from build123d import *

# Parameters (mm, degrees)
F1_DEPTH    = 1
F2_DEPTH    = 9
F2_TAPER    = 27
F3_T1_DEPTH = 17.6431556895
F3_T3_DEPTH = 17.6431556895
F3_T5_DEPTH = 17.6431556895
F3_T7_DEPTH = 17.6431556895
F4_R        = 18
F5_DEPTH    = 6
F5_TAPER    = 27
F6_R        = 3.05
F7_DEPTH    = 4.0010001


# Not quite as in the source:
# - a fillet or chamfer that OpenCascade refuses, or shapes differently, is made with other operations: its cross-section is extruded or revolved along the edge and cut away or added


with BuildPart() as f1:
    # F0 (on Top) → F1 (new body)
    with BuildSketch(Plane.XY):
        with BuildLine():
            Line((-17, -21), (17, -21))
            ThreePointArc((17, -21), (19.8284271247, -19.8284271247), (21, -17))
            Line((21, -17), (21, 17))
            ThreePointArc((21, 17), (19.8284271247, 19.8284271247), (17, 21))
            Line((17, 21), (-17, 21))
            ThreePointArc((-17, 21), (-19.8284271247, 19.8284271247), (-21, 17))
            Line((-21, 17), (-21, -17))
            ThreePointArc((-21, -17), (-19.8284271247, -19.8284271247), (-17, -21))
        make_face()
    extrude(amount=F1_DEPTH)

    # F1_face (on face) → F2 (join)
    with BuildSketch(Plane.XY.offset(1)):
        with BuildLine():
            Line((-17, -21), (17, -21))
            ThreePointArc((17, -21), (19.8284271247, -19.8284271247), (21, -17))
            Line((21, -17), (21, 17))
            ThreePointArc((21, 17), (19.8284271247, 19.8284271247), (17, 21))
            Line((17, 21), (-17, 21))
            ThreePointArc((-17, 21), (-19.8284271247, 19.8284271247), (-21, 17))
            Line((-21, 17), (-21, -17))
            ThreePointArc((-21, -17), (-19.8284271247, -19.8284271247), (-17, -21))
        make_face()
    extrude(amount=F2_DEPTH, taper=F2_TAPER)

    # F3: fillet of radius 4 on 4 edges, made by hand

    # F3_s2 → F3_t1 (cut)
    with BuildSketch(Plane(origin=(-6.1956825311, -6.1956825311, -12.1597116243), x_dir=(-0.7071067812, 0.7071067812, 0), z_dir=(0.4133841097, 0.4133841097, 0.8113119965))):
        with BuildLine():
            ThreePointArc((-2.5201470213, 22.6347249075), (0, 23.5284636515), (2.5201470213, 22.6347249075))
            Line((2.5201470213, 22.6347249075), (0, 24.6793504189))
            Line((0, 24.6793504189), (-2.5201470213, 22.6347249075))
        make_face()
    extrude(amount=F3_T1_DEPTH, mode=Mode.SUBTRACT)

    # F3_s4 → F3_t3 (cut)
    with BuildSketch(Plane(origin=(6.1956825311, -6.1956825311, -12.1597116243), x_dir=(-0.7071067812, -0.7071067812, 0), z_dir=(-0.4133841097, 0.4133841097, 0.8113119965))):
        with BuildLine():
            ThreePointArc((2.5201470213, 22.6347249075), (0, 23.5284636515), (-2.5201470213, 22.6347249075))
            Line((-2.5201470213, 22.6347249075), (0, 24.6793504189))
            Line((0, 24.6793504189), (2.5201470213, 22.6347249075))
        make_face()
    extrude(amount=F3_T3_DEPTH, mode=Mode.SUBTRACT)

    # F3_s6 → F3_t5 (cut)
    with BuildSketch(Plane(origin=(-6.1956825311, 6.1956825311, -12.1597116243), x_dir=(0.7071067812, 0.7071067812, 0), z_dir=(0.4133841097, -0.4133841097, 0.8113119965))):
        with BuildLine():
            ThreePointArc((-2.5201470213, 22.6347249075), (0, 23.5284636515), (2.5201470213, 22.6347249075))
            Line((2.5201470213, 22.6347249075), (0, 24.6793504189))
            Line((0, 24.6793504189), (-2.5201470213, 22.6347249075))
        make_face()
    extrude(amount=F3_T5_DEPTH, mode=Mode.SUBTRACT)

    # F3_s8 → F3_t7 (cut)
    with BuildSketch(Plane(origin=(6.1956825311, 6.1956825311, -12.1597116243), x_dir=(0.7071067812, -0.7071067812, 0), z_dir=(-0.4133841097, -0.4133841097, 0.8113119965))):
        with BuildLine():
            ThreePointArc((2.5201470213, 22.6347249075), (0, 23.5284636515), (-2.5201470213, 22.6347249075))
            Line((-2.5201470213, 22.6347249075), (0, 24.6793504189))
            Line((0, 24.6793504189), (2.5201470213, 22.6347249075))
        make_face()
    extrude(amount=F3_T7_DEPTH, mode=Mode.SUBTRACT)

    # F4 (on face) → F5 (cut)
    with BuildSketch(Plane(origin=(0, 0, 0), x_dir=(1, 0, 0), z_dir=(0, 0, -1))):
        Circle(F4_R)
    extrude(amount=-F5_DEPTH, taper=F5_TAPER, mode=Mode.SUBTRACT)

    # F6 (on face) → F7 (cut, through all)
    with BuildSketch(Plane(origin=(0, 0, 6), x_dir=(1, 0, 0), z_dir=(0, 0, -1))):
        Circle(F6_R)
    extrude(amount=-F7_DEPTH, mode=Mode.SUBTRACT)


solid = f1.part
Part model, mm, in its own coordinate system. A direction names the side the tool comes from. Give positions to 0.01 mm unless a question says otherwise; leave off trailing zeros. Order: outer loops, then holes, each group sorted by start corner. A loop starts at its lowest first (then second) coordinate and runs counter-clockwise, first axis right, second up. Notation, with made-up numbers: (5, 33.25) -> (54, 33.25) arc R33 ccw to (54, 61.25) -> close; hole circle Ø8 at (19, 74.5). An arc over 180 degrees is marked (long way). Use one line per item in the form item = value.
(1) Flat gauge pins, fed straight in: P1, Ø1.5, axis at x = -2, z = 8.5, coming from the -Y side; P2, Ø1, axis at y = -5, z = 6.5, coming from the -X side; P3, Ø5, axis at y = 3, z = 6, coming from the -X side; P4, Ø5, axis at x = 0, y = 0, coming from the +Z side (1 decimal). Where does each tip first touch, or does it go through?
Solution:
P1 = -17.56
P2 = -18.45
P3 = -19.73
P4 = through
(2) Pull direction Y, two halves, no side cores. Call faces 1 (the face through (-3.27, 14.73, 5.71)), 2 (the face through (-19.605, -19.548, 1.698)), 3 (the face through (18.739, 0.238, 5.437)), 4 (the face through (-3.047, -0.134, 7.972)): +Y half, -Y half, draft (parallel to the pull), parting line (faces both ways), or undercut.
Solution:
face_1 = undercut
face_2 = -Y half
face_3 = draft
face_4 = undercut
(3) Drill centre lines: line 1 (Z direction, x = -5.5, y = -15.5); line 2 (X direction, y = 1, z = 3.5); line 3 (Z direction, x = -1.5, y = 9). Where is each one in solid material? Low to high. Write a range as from..to.
Solution:
line_1 = 3.05..10
line_2 = -19.73..-16.19, 16.19..19.73
line_3 = 6..10
(4) Saw through at A-A (x = 0). Write the cut outline in (y, z), then the cut area to 3 significant figures.
Solution:
outline = (-21, 0) -> (-18, 0) -> (-14.94, 6) -> (-3.05, 6) -> (-3.05, 10) -> (-16.41, 10) -> (-21, 1) -> close; (3.05, 6) -> (14.94, 6) -> (18, 0) -> (21, 0) -> (21, 1) -> (16.41, 10) -> (3.05, 10) -> close
area = 157 mm²
(5) Tool access for faces 5 (the face through (0, -4, 6)), 6 (the face through (19.797, -19.859, 0.493)): list every direction of +Z, -Z, +X, -X, +Y, -Y with a clear straight run to the whole face (end or side of a thin tool).
Solution:
face_5 = -Z
face_6 = +Z, -Z, +X, -Y
